The figure shows three views and two pictorial views of one solid part (mm, origin at its lowest corner). Answer the questions. Round coordinates to 2 decimals unless told otherwise and drop trailing zeros. Loops run counter-clockwise (first coordinate to the right, second up) from the corner with the lowest first, then second, coordinate; pieces in that order, holes last. Notation, with made-up numbers: (-30.75, -15.5) -> (14.25, -15.5) arc R21 cw to (14.25, 18.5) -> close; hole circle Ø6 at (40.25, 42). An arc over 180 degrees is marked (long way). Write item = value, one per line. Start each with the question number.
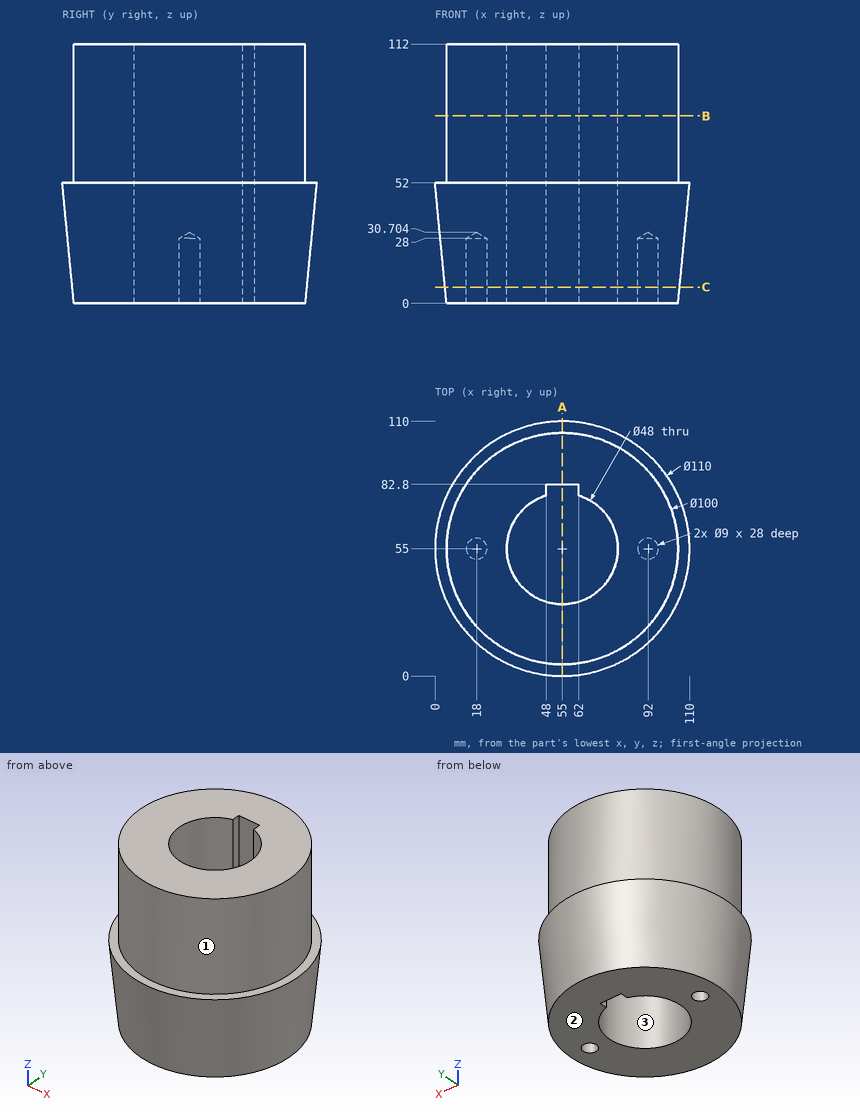
Item 1: Section C-C (z = 7) is taken. Determine the outline of the cut face in (x, y).
Item 2: The mould has two halves that part along X. Classify the marked faces 1, 2 and 3: pulls with the +X half, pulls with the -X half, needs draft (parallel to the pull), parting line crosses it, or undercut.
Item 3: Flat-ended cylindrical pins translate along their axes: pin 1 (4 mm diameter, centred on x = 86.5, z = 93.5, fed in from -Y); pin 2 (1.5 mm diameter, centred on y = 97, z = 38, fed in from -X); pin 3 (2.5 mm diameter, centred on y = 81.5, z = 74, fed in from +X). Find the tip coordinate at first contact, or state that the pin passes through.
Item 4: Find the intervals of material crossed by line 1 along X through (y, z) = (55, 25.5); line 2 along X through (y, z) = (55, 18); line 3 along Y through (x, z) = (33, 86), in increasing order. Write a range as [from, to].
Item 5: Section A-A (x = 55) is taken. Determine the outline of the cut face in (y, z), then the cut area to 3 significant figures.
Item 6: Section B-B (z = 81) is taken. Determine the outline of the cut face in (x, y), then the cut area to 3 significant figures.
Worked answers:
q1.outline = circle Ø101.35 at (55, 55); hole circle Ø9 at (18, 55); hole (48, 77.96) arc R24 ccw (long way) to (62, 77.96) -> (62, 82.8) -> (48, 82.8) -> close; hole circle Ø9 at (92, 55)
q2.face_1 = parting line crosses it
q2.face_2 = needs draft
q2.face_3 = undercut
q3.pin_1 = 14.63
q3.pin_2 = 20.68
q3.pin_3 = 98.16
q4.line_1 = [2.55, 13.5], [22.5, 31], [79, 87.5], [96.5, 107.45]
q4.line_2 = [3.27, 13.5], [22.5, 31], [79, 87.5], [96.5, 106.73]
q4.line_3 = [10.1, 45.41], [64.59, 99.9]
q5.outline = (0, 52) -> (5, 0) -> (31, 0) -> (31, 112) -> (5, 112) -> (5, 52) -> close; (82.8, 0) -> (105, 0) -> (110, 52) -> (105, 52) -> (105, 112) -> (82.8, 112) -> close
q5.area = 5,660 mm2
q6.outline = circle Ø100 at (55, 55); hole (48, 77.96) arc R24 ccw (long way) to (62, 77.96) -> (62, 82.8) -> (48, 82.8) -> close
q6.area = 5,990 mm2
